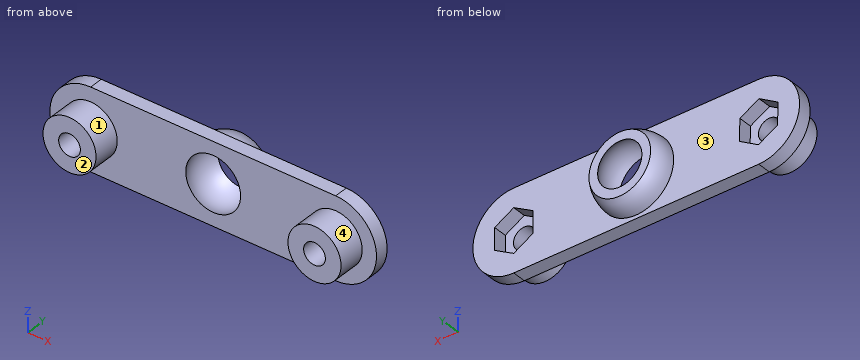
```python
from build123d import *
from build123d.topology import SkipClean

# Parameters (mm, degrees)
SKETCH1_R           = 1.6
SKETCH1_R_2         = 4.5
BOSS_EXTRUDE1_DEPTH = 2
BOSS_EXTRUDE2_START = 4
SKETCH2_R           = 3.9
SKETCH2_R_2         = 1.6
BOSS_EXTRUDE2_DEPTH = 4
CUT_EXTRUDE1_DEPTH  = 2


with BuildPart() as part:
    # Sketch1 → Boss-Extrude1 (new body)
    with BuildSketch(Plane(origin=(0, 0, 0), x_dir=(1, 0, 0), z_dir=(0, 1, 0))):
        with BuildLine():
            Line((-18, 6), (18, 6))
            ThreePointArc((18, 6), (24, 0), (18, -6))
            Line((18, -6), (-18, -6))
            ThreePointArc((-18, -6), (-24, 0), (-18, 6))
        make_face()
        with Locations(Location((18, 0, 0), (0, 0, 270))):
            Circle(SKETCH1_R, mode=Mode.SUBTRACT)
        with Locations(Location((-18, 0, 0), (0, 0, 90))):
            Circle(SKETCH1_R, mode=Mode.SUBTRACT)
        with Locations(Location((0, 0, 0), (0, 0, 270))):
            Circle(SKETCH1_R_2, mode=Mode.SUBTRACT)
    extrude(amount=BOSS_EXTRUDE1_DEPTH)

    # Sketch2 → Boss-Extrude2 (add)
    # profile 1 of 2: a face of its own
    with SkipClean():  # the faces are left unmerged after this step: merging them gives an invalid solid
        with BuildSketch(Plane.XZ.offset(BOSS_EXTRUDE2_START)):
            with Locations(Location((-18, 0, 0), (0, 0, 90))):
                Circle(SKETCH2_R)
            with Locations(Location((-18, 0, 0), (0, 0, 270))):
                Circle(SKETCH2_R_2, mode=Mode.SUBTRACT)
        # profile 2 of 2: a face of its own
        with BuildSketch(Plane.XZ.offset(BOSS_EXTRUDE2_START)):
            with Locations(Location((18, 0, 0), (0, 0, 90))):
                Circle(SKETCH2_R)
            with Locations(Location((18, 0, 0), (0, 0, 270))):
                Circle(SKETCH2_R_2, mode=Mode.SUBTRACT)
        extrude(amount=-BOSS_EXTRUDE2_DEPTH)

    # Sketch3 → Revolve1 (revolve)
    with SkipClean():  # the faces are left unmerged after this step: merging them gives an invalid solid
        with BuildSketch(Plane(origin=(0, 0, 0), x_dir=(0, 0, -1), z_dir=(1, 0, 0))):
            with BuildLine():
                Line((-3.25, 5.112474899), (-4.534589287, 5.112474899))
                ThreePointArc((-4.534589287, 5.112474899), (-5.463872545, 2.629362224), (-5.123475383, 0))
                Line((-5.123475383, 0), (-4.031128874, 0))
                ThreePointArc((-4.031128874, 0), (-4.448377156, 2.679662181), (-3.25, 5.112474899))
            make_face()
            with BuildLine():
                Line((3.25, 5.112474899), (4.534589287, 5.112474899))
                ThreePointArc((4.534589287, 5.112474899), (5.463872545, 2.629362224), (5.123475383, 0))
                Line((5.123475383, 0), (4.031128874, 0))
                ThreePointArc((4.031128874, 0), (4.448377156, 2.679662181), (3.25, 5.112474899))
            make_face()
        revolve(axis=Axis((0, 5.800326489, 0), (0, -1, 0)))

    # Sketch4 → Cut-Extrude1 (cut)
    with BuildSketch(Plane(origin=(0, 2, 0), x_dir=(1, 0, 0), z_dir=(0, 1, 0))):
        Polygon((-15.227114181, -1.662659787), (-15.173651477, 1.570059667), (-17.946537296, 3.232719455), (-20.772885819, 1.662659787), (-20.826348523, -1.570059667), (-18.053462704, -3.232719455), align=None)
        Polygon((18, -3.233161507), (20.8, -1.616580754), (20.8, 1.616580754), (18, 3.233161507), (15.2, 1.616580754), (15.2, -1.616580754), align=None)
    extrude(amount=-CUT_EXTRUDE1_DEPTH, mode=Mode.SUBTRACT)


solid = part.part
```
For this review, take the finished solid that the model builds, in its own axes (mm). Face numbers are marked on the shaded views. A direction names the side the tool comes from. Round coordinates to 2 decimals unless told otherwise and drop trailing zeros. Write each loop counter-clockwise with the first axis right and the second up, starting at its lowest first coordinate (ties: lowest second). Pieces come first, ordered by that corner, then holes. Notation, with made-up numbers: (-6, 23.5) -> (27, 23.5) arc R17 ccw to (27, 55.5) -> close; hole circle Ø5 at (42, 33.25). An arc over 180 degrees is marked (long way). Use one line per item in the form item = value.
Q1. Machinability: for the marked faces 1 and 2, which of the approach directions +Z, -Z, +X, -X, +Y, -Y give a long, thin tool a straight path to every point of the face, cutting with its end or side? Answer none if there is none.
Resolved:
face_1 = -Y
face_2 = +Z, -Z, +X, -X, -Y
Q2. Consider section A-A (y = -2). State the section outline as (x, z) points.
Resolved:
outline = circle Ø7.8 at (-18, 0); circle Ø7.8 at (18, 0); hole circle Ø3.2 at (-18, 0); hole circle Ø3.2 at (18, 0)
Q3. Clearance check with flat-ended pins moving along their axes: pin 1 Ø3.5 at (x, z) = (4, 0.5) entering from -Y; pin 2 Ø4 at (x, z) = (-18, 0) entering from +Y; pin 3 Ø4 at (x, z) = (18, -4) entering from +Y. State where each tip first meets the part, or that it passes through.
Resolved:
pin_1 = 0
pin_2 = 0
pin_3 = 2
Q4. The part is to be moulded in two halves that separate along X. For the marked faces 3 and 4, say which applies: released by +X, released by -X, zero draft, split by the parting line, or undercut.
Resolved:
face_3 = zero draft
face_4 = undercut
Q5. To check wall thickness, follow probe 1 along X at (y, z) = (-3.05, 0); probe 2 along Z at (x, y) = (-18, -3.05); probe 3 along Y at (x, z) = (14.5, -2.75). State the ranges of each line that lie inside material, in increasing order. Write a range as from..to.
Resolved:
probe_1 = -21.9..-19.6, -16.4..-14.1, 14.1..16.4, 19.6..21.9
probe_2 = -3.9..-1.6, 1.6..3.9
probe_3 = 0..2
Q6. Consider section B-B (z = 2.5). State the section outline as (x, y) points.
Resolved:
outline = (-23.45, 0) -> (-20.99, 0) -> (-20.99, -4) -> (-15.01, -4) -> (-15.01, 0) -> (-3.16, 0) arc R3.74 cw to (-2.08, 5.11) -> (-3.78, 5.11) arc R4.9 ccw to (-4.9, 2) -> (-16.73, 2) -> (-16.73, 0) -> (-19.28, 0) -> (-19.28, 2) -> (-23.45, 2) -> close; (2.08, 5.11) arc R3.74 cw to (3.16, 0) -> (15.01, 0) -> (15.01, -4) -> (20.99, -4) -> (20.99, 0) -> (23.45, 0) -> (23.45, 2) -> (19.27, 2) -> (19.27, 0) -> (16.73, 0) -> (16.73, 2) -> (4.9, 2) arc R4.9 ccw to (3.78, 5.11) -> close
Q7. Consider section C-C (x = 19). State the section outline as (y, z) points.
Resolved:
outline = (-4, -3.77) -> (0, -3.77) -> (0, -5.92) -> (2, -5.92) -> (2, -2.66) -> (0, -2.66) -> (0, -1.25) -> (-4, -1.25) -> close; (-4, 1.25) -> (0, 1.25) -> (0, 2.66) -> (2, 2.66) -> (2, 5.92) -> (0, 5.92) -> (0, 3.77) -> (-4, 3.77) -> close
Q8. Consider section D-D (y = 1). State the section outline as (x, z) points, then the cut area to 3 significant figures.
Resolved:
outline = (-18, -6) -> (18, -6) arc R6 ccw to (18, 6) -> (-18, 6) arc R6 ccw to start; hole (-20.83, 1.57) -> (-20.77, -1.66) -> (-17.95, -3.23) -> (-15.17, -1.57) -> (-15.23, 1.66) -> (-18.05, 3.23) -> close; hole circle Ø8.77 at (0, 0); hole (15.2, -1.62) -> (18, -3.23) -> (20.8, -1.62) -> (20.8, 1.62) -> (18, 3.23) -> (15.2, 1.62) -> close
area = 430 mm²
